Verification items for the finished model (mm, model axes). Face numbers are marked on the shaded views. A direction names the side the tool comes from. Give positions to 0.01 mm unless a question says otherwise; leave off trailing zeros. Write each loop counter-clockwise with the first axis right and the second up, starting at its lowest first coordinate (ties: lowest second). Pieces come first, ordered by that corner, then holes. Notation, with made-up numbers: (40.5, 31) - (46.5, 31) arc R29 ccw to (46.5, 65) - close; hole circle Ø4 at (43.5, -11.5). An arc over 180 degrees is marked (long way). Answer as a JSON object with one key per item and string values. Group by question number.
Item 1: Tool access check on the marked faces 1, 2, 3 and 4. Record the directions out of +Z, -Z, +X, -X, +Y, -Y that give a thin tool (end or side, any length) a straight path to the whole face; none if there is none.
Item 2: Sectioned sample at B-B, the plane x = 106. Record the boundary of the cut face in (y, z).
Item 3: Sectioned sample at C-C, the plane y = -60. Record the boundary of the cut face in (x, z), and give its area (3 significant figures).
Item 4: Draft check along Y on the marked faces 5, 6 and 7. Enter one of: +Y half, -Y half, draft (parallel to the pull), parting line (faces both ways), or undercut.
Item 5: Scan lines: line 1 along X through (y, z) = (-21, 32); line 2 along Y through (x, z) = (106, 6); line 3 along Z through (x, y) = (99, -28). Record each from-to range of solid material in increasing order. Write a range as [from, to].
Item 6: Go/stop test with flat-tipped pins: pin 1 (12 mm diameter, centred on x = 131.5, y = -33, fed in from -Z); pin 2 (1.5 mm diameter, centred on y = -44.5, z = 5, fed in from -X); pin 3 (12.5 mm diameter, centred on y = -19.5, z = 34.5, fed in from -X); pin 4 (10 mm diameter, centred on y = -59, z = 14.5, fed in from +X). Record where each tip stops, or that it passes through.
Item 7: Sectioned sample at A-A, the plane y = -33. Record the boundary of the cut face in (x, z), and give its area (3 significant figures).
Item 8: Sectioned sample at D-D, the plane z = 18. Record the boundary of the cut face in (x, y), and give its area (3 significant figures).
```python
from build123d import *

# Parameters (mm, degrees)
F1_DEPTH      = 66
F3_DEPTH      = 72.501
F4_W          = 25
F4_H          = 25
F5_DEPTH      = 50
F5_DEPTH_BACK = 142
F6_R          = 7.5
F7_DEPTH      = 25.001
F8_R          = 5
F9_DEPTH      = 25
F10_R         = 8
F11_W         = 12
F11_H         = 25
F12_DEPTH     = 5
F14_D         = 3


with BuildPart() as f1:
    # F0 (on Front) → F1 (new body)
    with BuildSketch(Plane.XZ):
        Polygon((0, 25), (0, 0), (92, 0), (92, 25), (72.5, 25), (72.5, 50), (19.5, 50), (19.5, 25), align=None)
    extrude(amount=F1_DEPTH)

    # F2 (on face) → F3 (cut, through all)
    with BuildSketch(Plane.YZ.offset(72.5)):
        Polygon((-62.5, 50), (-66, 50), (-66, 46.5), align=None)
        Polygon((0, 46.5), (0, 50), (-3.5, 50), align=None)
    extrude(amount=-F3_DEPTH, mode=Mode.SUBTRACT)

    # F4 (on face) → F5 (join, two sides)
    with BuildSketch(Plane.YZ.offset(92)) as f5_sk:
        with Locations((-33, 12.5)):
            Rectangle(F4_W, F4_H)
    extrude(amount=F5_DEPTH)
    extrude(f5_sk.sketch, amount=-F5_DEPTH_BACK)

    # F6 (on face) → F7 (cut, through all)
    with BuildSketch(Plane.XY.offset(25)):
        with Locations((131.5, -33)):
            Circle(F6_R)
        with Locations((-39.5, -33)):
            Circle(F6_R)
    extrude(amount=-F7_DEPTH, mode=Mode.SUBTRACT)

    # F8 (on face) → F9 (cut)
    with BuildSketch(Plane.XY.offset(25)):
        with Locations((106, -33)):
            Circle(F8_R)
    extrude(amount=-F9_DEPTH, mode=Mode.SUBTRACT)

    # F10
    f10_edges = [f1.edges().sort_by_distance(p)[0] for p in [
        (142, -20.5, 12.5),
        (142, -45.5, 12.5),
        (-50, -45.5, 12.5),
        (-50, -20.5, 12.5),
    ]]
    fillet(f10_edges, radius=F10_R)

    # F11 (on face) → F12 (cut)
    with BuildSketch(Plane.XY.offset(25)):
        with Locations((106, -33)):
            Rectangle(F11_W, F11_H)
    extrude(amount=-F12_DEPTH, mode=Mode.SUBTRACT)

    # F14 (through all)
    with Locations(Plane.XZ.offset(66)):
        with Locations((28.5, 32.5), (63.5, 32.5), (63.5, 9), (28.5, 9)):
            Hole(F14_D / 2)


solid = f1.part
```
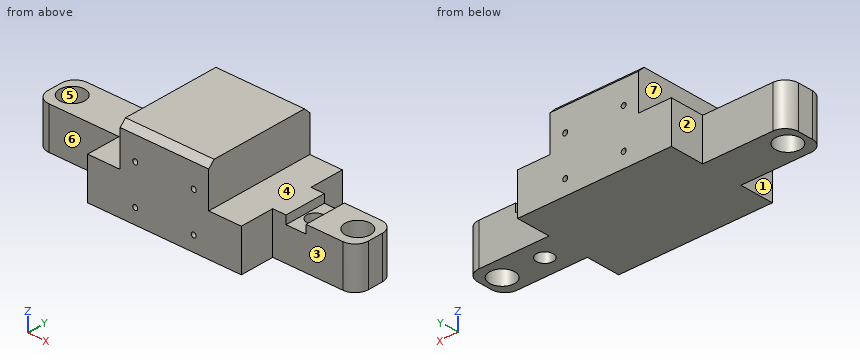
Geometry check:
{
 "1": {"face 1": "+Z, -Z, -X, -Y", "face 2": "+Z, -Z, -X, +Y", "face 3": "+Z, -Z, +X, -Y", "face 4": "+Z, +X, +Y, -Y"},
 "2": {"outline": "(-45.5, 0) - (-38, 0) - (-38, 20) - (-45.5, 20) - close; (-28, 0) - (-20.5, 0) - (-20.5, 20) - (-28, 20) - close"},
 "3": {"outline": "(0, 0) - (92, 0) - (92, 25) - (72.5, 25) - (72.5, 50) - (19.5, 50) - (19.5, 25) - (0, 25) - close; hole circle Ø3 at (28.5, 9); hole circle Ø3 at (28.5, 32.5); hole circle Ø3 at (63.5, 9); hole circle Ø3 at (63.5, 32.5)", "area": "3,600 mm^2"},
 "4": {"face 5": "undercut", "face 6": "-Y half", "face 7": "draft"},
 "5": {"line 1": "[19.5, 27.09], [29.91, 62.09], [64.91, 72.5]", "line 2": "[-45.5, -38], [-28, -20.5]", "line 3": "[0, 25]"},
 "6": {"pin 1": "through", "pin 2": "x = -46.99", "pin 3": "x = 19.5", "pin 4": "x = 92"},
 "7": {"outline": "(-50, 0) - (-47, 0) - (-47, 25) - (-50, 25) - close; (-32, 0) - (101, 0) - (101, 20) - (100, 20) - (100, 25) - (72.5, 25) - (72.5, 50) - (19.5, 50) - (19.5, 25) - (-32, 25) - close; (111, 0) - (124, 0) - (124, 25) - (112, 25) - (112, 20) - (111, 20) - close; (139, 0) - (142, 0) - (142, 25) - (139, 25) - close; hole circle Ø3 at (28.5, 9); hole circle Ø3 at (28.5, 32.5); hole circle Ø3 at (63.5, 9); hole circle Ø3 at (63.5, 32.5)", "area": "5,090 mm^2"},
 "8": {"outline": "(-50, -37.5) arc R8 ccw to (-42, -45.5) - (0, -45.5) - (0, -66) - (92, -66) - (92, -45.5) - (134, -45.5) arc R8 ccw to (142, -37.5) - (142, -28.5) arc R8 ccw to (134, -20.5) - (92, -20.5) - (92, 0) - (0, 0) - (0, -20.5) - (-42, -20.5) arc R8 ccw to (-50, -28.5) - close; hole circle Ø15 at (-39.5, -33); hole circle Ø10 at (106, -33); hole circle Ø15 at (131.5, -33)", "area": "8,090 mm^2"}
}
